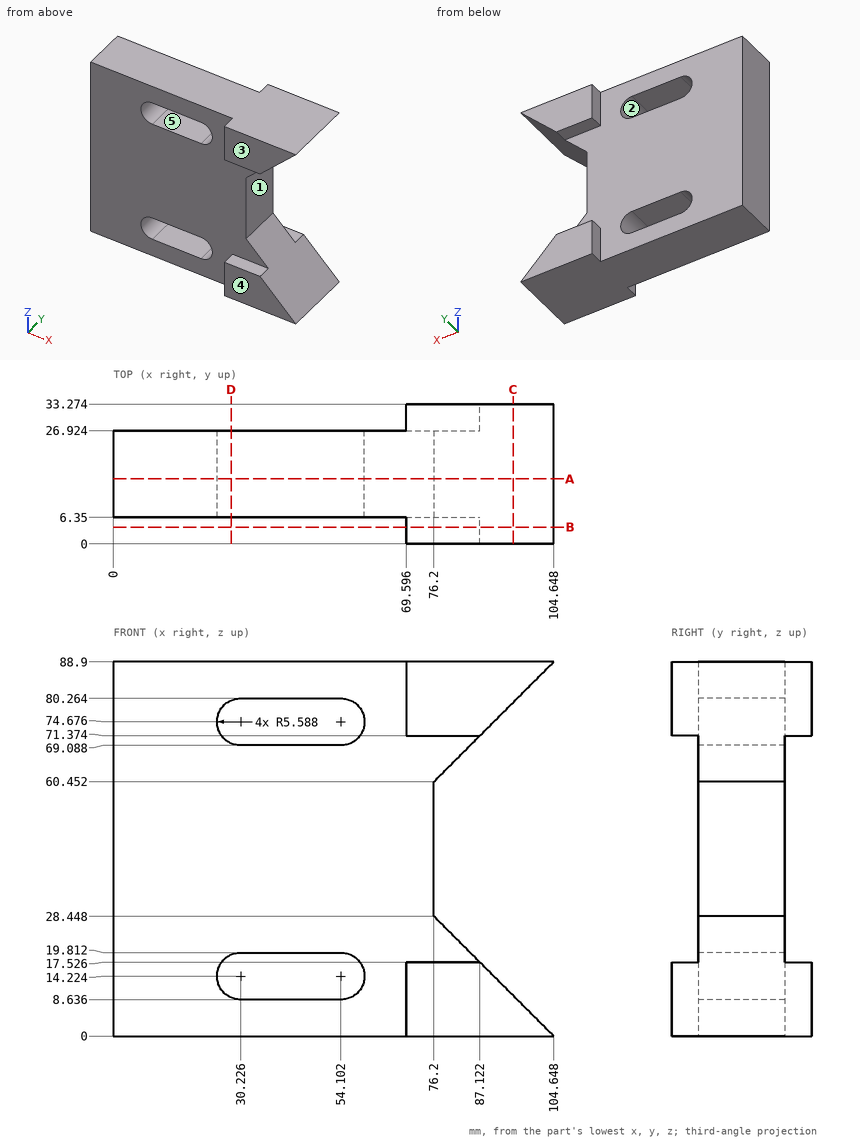
Design review of the part shown in the three views and the two pictorial views. Dimensions are in mm from the part's minimum x, y and z. A direction names the side the tool comes from. Coordinates: 2 decimals unless noted, no trailing zeros. Loops run counter-clockwise (first coordinate to the right, second up) from the corner with the lowest first, then second, coordinate; pieces in that order, holes last.
Q1. The part is to be moulded in two halves that separate along X. For the marked faces 1, 2 and 3, say which applies: +X half, -X half, draft (parallel to the pull), parting line (faces both ways), or undercut.
Reported:
face 1: +X half
face 2: undercut
face 3: draft
Q2. To check wall thickness, follow line 1 (Z direction, x = 51, y = 14); line 2 (Z direction, x = 79, y = 4.5); line 3 (Y direction, x = 58.5, z = 64.5). State the ranges of each line that lie inside material, in increasing order.
Reported:
line 1: z = 0 to 8.64, 19.81 to 69.09, 80.26 to 88.9
line 2: z = 0 to 17.53, 71.37 to 88.9
line 3: y = 6.35 to 26.92
Q3. We need section B-B on y = 4. State the section outline as (x, z) points.
Reported:
outline: (69.6, 0) - (104.65, 0) - (87.12, 17.53) - (69.6, 17.53) - close; (69.6, 71.37) - (87.12, 71.37) - (104.65, 88.9) - (69.6, 88.9) - close
Q4. We need section C-C on x = 95. State the section outline as (y, z) points, and give its area (3 significant figures).
Reported:
outline: (0, 0) - (33.27, 0) - (33.27, 9.65) - (0, 9.65) - close; (0, 79.25) - (33.27, 79.25) - (33.27, 88.9) - (0, 88.9) - close
area: 642 mm2
Q5. We need section A-A on y = 15.5. State the section outline as (x, z) points, and give its area (3 significant figures).
Reported:
outline: (0, 0) - (104.65, 0) - (76.2, 28.45) - (76.2, 60.45) - (104.65, 88.9) - (0, 88.9) - close; hole (30.23, 8.64) - (54.1, 8.64) arc R5.59 ccw to (54.1, 19.81) - (30.23, 19.81) arc R5.59 ccw to start; hole (30.23, 69.09) - (54.1, 69.09) arc R5.59 ccw to (54.1, 80.26) - (30.23, 80.26) arc R5.59 ccw to start
area: 6,850 mm2
Q6. We need section D-D on x = 28. State the section outline as (y, z) points, and give its area (3 significant figures).
Reported:
outline: (6.35, 0) - (26.92, 0) - (26.92, 9.1) - (6.35, 9.1) - close; (6.35, 19.35) - (26.92, 19.35) - (26.92, 69.55) - (6.35, 69.55) - close; (6.35, 79.8) - (26.92, 79.8) - (26.92, 88.9) - (6.35, 88.9) - close
area: 1,410 mm2
Q7. For pin 1 (3 mm diameter, centred on y = 31, z = 76, fed in from -X); pin 2 (10 mm diameter, centred on x = 82.5, z = 58.5, fed in from -Y); pin 3 (5 mm diameter, centred on x = 15, z = 28.5, fed in from +Y); pin 4 (10.5 mm diameter, centred on y = 18, z = 37, fed in from +X), all flat-tipped, find the tip position at first contact; note any pin that passes through.
Reported:
pin 1: stops at x = 69.6
pin 2: passes through
pin 3: stops at y = 26.92
pin 4: stops at x = 76.2
Q8. Tool access review of the marked faces 4 and 5: name each direction out of +Z, -Z, +X, -X, +Y, -Y from which nothing blocks a thin tool from reaching the whole face with its end or side.
Reported:
face 4: +Z, -Z, +X, -X, -Y
face 5: +Y, -Y
